Can you work these out from the model? Positions are in its coordinate system, mm. Coordinates: 2 decimals unless noted, no trailing zeros. Loops run counter-clockwise (first coordinate to the right, second up) from the corner with the lowest first, then second, coordinate; pieces in that order, holes last. Notation, with made-up numbers: (88.5, -11) -> (122.5, -11) arc R16 ccw to (122.5, -5) -> close; hole circle Ø2 at (78, 6). An arc over 180 degrees is marked (long way). Use one line per item in the form item = value. Start each with the question number.
(1) I'm going to push a flat-ended pin straight in: pin 1 (0.6 mm diameter, centred on x = 285.5, y = 1, fed in from -Z). Where does the tip first touch, or does it pass through?
(2) I need wall thicknesses on line 1 (Z direction, x = 354, y = 1.4); line 2 (X direction, y = 0.1, z = -21.5); line 3 (X direction, y = 1.75, z = -31). Which ranges of each line are inside material? Lowest first, please. Write a range as [from, to].
(3) Imagine slicing it at A-A (x = 203.5). List the corners of the cut face in (y, z) for me.
Autodesk Fusion 360 part; units mm, degrees
sketch "Sketch1" plane through (0, 0, 0) normal (0, 1, 0) x (1, 0, 0)
  line L0 (0, 0) -> (419.4969, 0)
  line L1 (419.4969, 0) -> (419.4969, 44.45)
  line L2 (419.4969, 44.45) -> (0, 44.45)
  line L3 (0, 44.45) -> (0, 0)
  line L4 (-8.9507, 43.45) -> (460, 43.45) construction
  line L5 (-8.9686, 29.45) -> (500, 29.45) construction
  line L6 (399.4969, 0) -> (399.4969, 44.45)
  line L7 (20, 44.45) -> (20, 0)
  line L8 (20, 29.45) -> (399.4969, 29.45)
  dimension "d1" = 419.4969
  dimension "d2" = 44.45
  dimension "d3" = 1
  dimension "d13" = 14
  dimension "d14" = 20
  dimension "d15" = 20
extrude "Extrude1" add sketch "Sketch1" along normal blind 2 contours L0 L2 L3 L7 | L0 L6 L7 L8 | L0 L1 L2 L6
sketch "Sketch2" plane through (419.4969, 0, 0) normal (1, 0, 0) x (0, 0, -1)
  line L0 (0, 0) -> (44.45, 0)
  line L1 (44.45, 0) -> (44.45, 2)
  line L2 (44.45, 2) -> (0, 2)
  line L3 (0, 2) -> (0, 0)
  line L4 (43.45, 0) -> (43.45, 2) construction
  circle A0 centre (43.45, 1) radius 1
  point P0 (43.45, 0)
extrude "Extrude2" add sketch "Sketch2" along normal blind 2 contours A0
extrude "Extrude3" add sketch "Sketch2" against normal blind 2 from surface at -419.4969 contours A0
chamfer "Chamfer1" distance 5 angle 45 1 edges at (419.4969, 1, 0)
chamfer "Chamfer1" distance 5 angle 45 1 edges at (0, 1, 0)
fillet "Fillet1" radius 10 4 edges at (399.4969, 1, -44.45) (399.4969, 1, -29.45) (20, 1, -29.45) (20, 1, -44.45)
equation "d1 = 16 33/64\""
equation "d2 = 1 3/4\""
equation "d15 = d14"
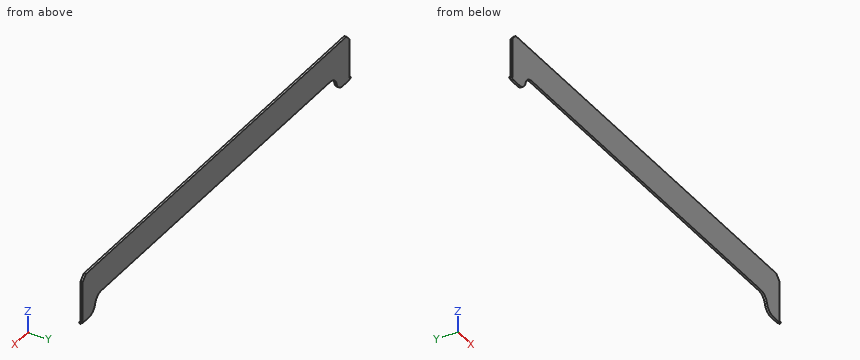
Worked out:
q1.pin_1 = -29.45
q2.line_1 = [-29.45, 0]
q2.line_2 = [0, 419.5]
q2.line_3 = [0, 24.65], [395.48, 419.5]
q3.outline = (0, -29.45) -> (2, -29.45) -> (2, 0) -> (0, 0) -> close
